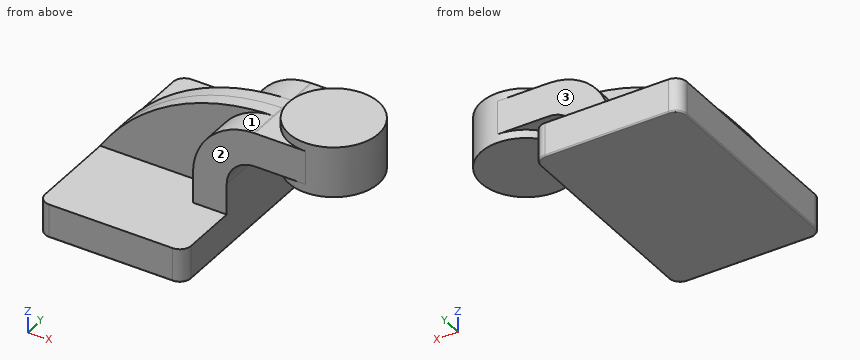
```python
from build123d import *

# Parameters (mm, degrees)
F1_DEPTH = 63.5
F0_W     = 25.4
F0_H     = 19.05
F2_DEPTH = 25.4
F3_DEPTH = 7.9375
F5_R     = 6.35
F6_R     = 0.762


with BuildPart() as f1:
    # F0 (on Front) → F1 (new body, symmetric)
    with BuildSketch(Plane.XZ):
        Polygon((41.275, -9.525), (41.275, 9.525), (22.225, 9.525), (-41.275, 9.525), (-41.275, -9.525), align=None)
    extrude(amount=F1_DEPTH, both=True)

    # F0 (on Front) → F2 (join, symmetric)
    with BuildSketch(Plane.XZ):
        with BuildLine():
            Line((22.225, 9.525), (41.275, 9.525))
            Line((41.275, 9.525), (41.275, 27.0002))
            ThreePointArc((41.275, 27.0002), (45.9246798487, 38.2255201513), (57.15, 42.8752))
            Line((57.15, 42.8752), (60.325, 42.8752))
            Line((60.325, 42.8752), (60.325, 61.9252))
            Line((60.325, 61.9252), (57.15, 61.9252))
            add(Edge.make_bspline(
                [(56.5144411646, 61.9194166288), (56.7262412244, 61.9218660962), (56.9380948845, 61.9237939637), (57.15, 61.9252)],
                knots=[110.8989098022, 110.8989098022, 110.8989098022, 110.8989098022, 111.5045361635, 111.5045361635, 111.5045361635, 111.5045361635], degree=3))
            ThreePointArc((56.5144411646, 61.9194166288), (32.2306047693, 51.4701686623), (22.225, 27.0002))
            Line((22.225, 27.0002), (22.225, 9.525))
        make_face()
        with Locations((73.025, 52.4002)):
            Rectangle(F0_W, F0_H)
    extrude(amount=F2_DEPTH, both=True)

    # F0 (on Front) → F3 (join, symmetric)
    with BuildSketch(Plane.XZ):
        with BuildLine():
            Line((-41.275, 9.525), (22.225, 9.525))
            Line((22.225, 9.525), (22.225, 27.0002))
            ThreePointArc((22.225, 27.0002), (32.2306047693, 51.4701686623), (56.5144411646, 61.9194166288))
            add(Edge.make_bspline(
                [(-41.275, 9.525), (-19.2555756955, 43.5326460608), (17.7307995872, 61.4708838699), (56.5144411646, 61.9194166288)],
                knots=[0, 0, 0, 0, 110.8989098022, 110.8989098022, 110.8989098022, 110.8989098022], degree=3))
        make_face()
    extrude(amount=F3_DEPTH, both=True)

    # F0 (on Front) → F4 (revolve)
    with BuildSketch(Plane.XZ):
        Polygon((85.725, 61.9252), (85.725, 42.8752), (85.725, 38.1), (111.125, 38.1), (111.125, 66.675), (85.725, 66.675), align=None)
    revolve(axis=Axis((85.725, 0, 52.3875), (0, 0, 1)))

    # F5
    f5_edges = [f1.edges().sort_by_distance(p)[0] for p in [
        (-41.275, -63.5, 0),
        (41.275, -63.5, 0),
        (41.275, 63.5, 0),
        (-41.275, 63.5, 0),
    ]]
    fillet(f5_edges, radius=F5_R)

    # F6
    f6_edges = [f1.edges().sort_by_distance(p)[0] for p in [
        (0, 63.5, -9.525),
        (-39.415128, 61.640128, -9.525),
        (39.415128, 61.640128, -9.525),
        (-41.275, 0, -9.525),
        (41.275, 0, -9.525),
        (-39.415128, -61.640128, -9.525),
        (39.415128, -61.640128, -9.525),
        (0, -63.5, -9.525),
    ]]
    fillet(f6_edges, radius=F6_R)


solid = f1.part
```
Input: part model. Units: mm. Frame: model coordinates. Face numbers are marked on the shaded views. A direction names the side the tool comes from. Give positions to 0.01 mm unless a question says otherwise; leave off trailing zeros. Write each loop counter-clockwise with the first axis right and the second up, starting at its lowest first coordinate (ties: lowest second). Pieces come first, ordered by that corner, then holes. Notation, with made-up numbers: (-6.75, 0.25) - (26.25, 0.25) arc R26 ccw to (26.25, 19.25) - close; hole circle Ø1 at (37.5, 10.5). An arc over 180 degrees is marked (long way). Write item = value, one per line. Start each with the question number.
1. Access query for the marked faces 1, 2 and 3. Directions: +Z, -Z, +X, -X, +Y, -Y. A direction counts if a zero-diameter tool reaches every point of the face in a straight line with its end or side. Return the directions, or none.
2. Ray query, L1, parallel to X at y = -39, z = 6 (3 decimals); L2, parallel to Z at x = -2, y = 51.5 (3 decimals); L3, parallel to X at y = 9, z = 17.5 (3 decimals). Return the intervals inside material, ascending.
3. First-contact query: pin 1 Ø5 at (x, z) = (-7.5, 49) entering from +Y; pin 2 Ø10 at (y, z) = (-11, 50) entering from -X; pin 3 Ø10.5 at (y, z) = (7.5, 7.5) entering from +X (3 decimals); pin 4 Ø16.5 at (x, y) = (4, 48) entering from +Z (3 decimals). Flat tips, straight axial feed; report the tip coordinate or a pass-through.
4. Section query A-A, the plane y = -40. Output: boundary loops of the cut face in (x, z) (3 decimals).
5. Section query B-B, the plane x = 72. Output: boundary loops of the cut face in (y, z) (3 decimals).
6. Section query C-C, the plane x = 97. Output: boundary loops of the cut face in (y, z) (3 decimals).
Check sheet entries:
q1.face_1 = +Z, -X, -Y
q1.face_2 = +Z, +X, -X, -Y
q1.face_3 = +Z, +X, -X, +Y
q2.L1 = -41.275 to 41.275
q2.L2 = -9.525 to 9.525
q2.L3 = 22.225 to 41.275
q3.pin_1 = through
q3.pin_2 = -2.79
q3.pin_3 = 41.275
q3.pin_4 = 9.525
q4.outline = (-41.275, -8.763) arc R0.762 ccw to (-40.513, -9.525) - (40.513, -9.525) arc R0.762 ccw to (41.275, -8.763) - (41.275, 9.525) - (-41.275, 9.525) - close
q5.outline = (-25.4, 42.875) - (-21.373, 42.875) - (-21.373, 38.1) - (21.373, 38.1) - (21.373, 42.875) - (25.4, 42.875) - (25.4, 61.925) - (21.373, 61.925) - (21.373, 66.675) - (-21.373, 66.675) - (-21.373, 61.925) - (-25.4, 61.925) - close
q6.outline = (-22.76, 38.1) - (22.76, 38.1) - (22.76, 66.675) - (-22.76, 66.675) - close
